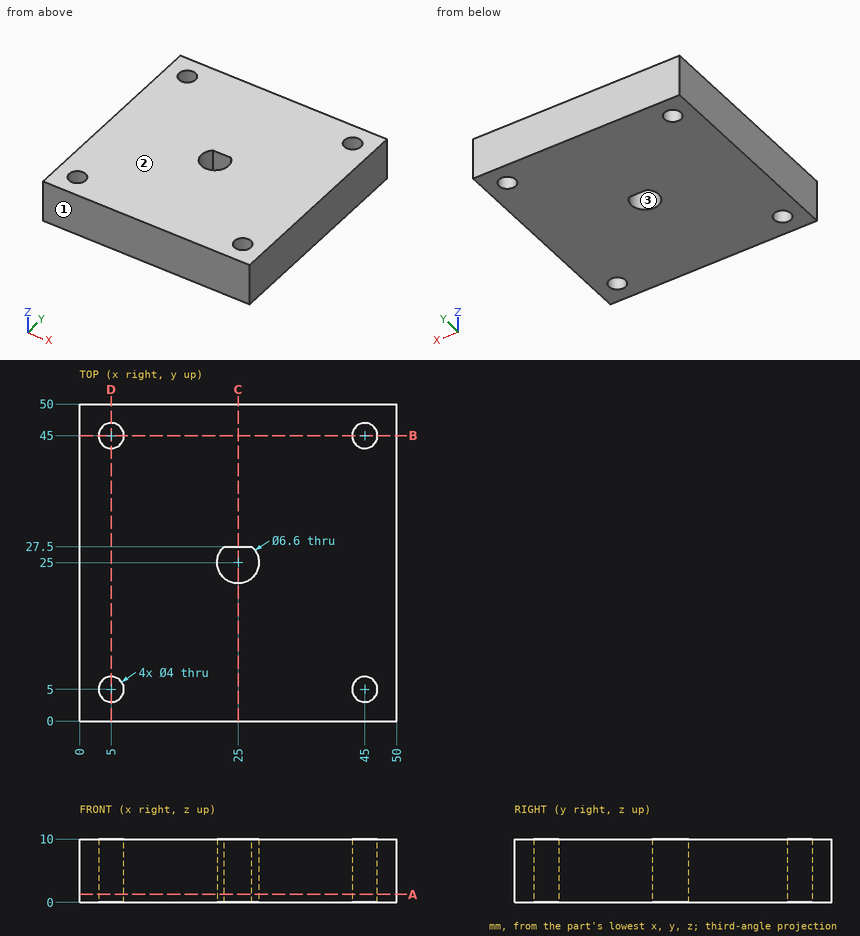
Job drawing, mm, ordinate dimensions from the low corner. One solid piece. Round coordinates to 2 decimals unless told otherwise and drop trailing zeros. Loops run counter-clockwise (first coordinate to the right, second up) from the corner with the lowest first, then second, coordinate; pieces in that order, holes last. Notation, with made-up numbers: (50.5, 8) -> (61.5, 8) arc R24 cw to (61.5, 39) -> close; hole circle Ø5 at (6.25, 44). An arc over 180 degrees is marked (long way). Use a Markdown table: item, result.
1) Drop flat-ended pins along their axis: pin 1 Ø3.5 at (x, y) = (45, 5) entering from -Z; pin 2 Ø12 at (x, y) = (26, 25.5) entering from +Z. Give the stop position or say it passes through.
The answers:
| item | result |
|---|---|
| pin 1 | passes through |
| pin 2 | stops at z = 10 |
2) Cut at C-C, the plane x = 25. List the corners of the cut face in (y, z).
The answers:
| item | result |
|---|---|
| outline | (0, 0) -> (21.7, 0) -> (21.7, 10) -> (0, 10) -> close; (27.5, 0) -> (50, 0) -> (50, 10) -> (27.5, 10) -> close |
3) Pull direction Y, two halves, no side cores. Call the marked faces 1, 2 and 3: pulls with the +Y half, pulls with the -Y half, needs draft (parallel to the pull), parting line crosses it, or undercut.
The answers:
| item | result |
|---|---|
| face 1 | pulls with the -Y half |
| face 2 | needs draft |
| face 3 | undercut |
4) Cut at A-A, the plane z = 1.25. List the corners of the cut face in (x, y).
The answers:
| item | result |
|---|---|
| outline | (0, 0) -> (50, 0) -> (50, 50) -> (0, 50) -> close; hole circle Ø4 at (5, 5); hole circle Ø4 at (5, 45); hole (22.85, 27.5) arc R3.3 ccw (long way) to (27.15, 27.5) -> close; hole circle Ø4 at (45, 5); hole circle Ø4 at (45, 45) |
5) Cut at B-B, the plane y = 45. List the corners of the cut face in (x, z).
The answers:
| item | result |
|---|---|
| outline | (0, 0) -> (3, 0) -> (3, 10) -> (0, 10) -> close; (7, 0) -> (43, 0) -> (43, 10) -> (7, 10) -> close; (47, 0) -> (50, 0) -> (50, 10) -> (47, 10) -> close |
6) Probe line 1 (Y direction, x = 5, z = 4.25); line 2 (X direction, y = 25, z = 3.5); line 3 (Y direction, x = 43.5, z = 7.25). List the from-to ranges inside material, lowest first. Write a range as [from, to].
The answers:
| item | result |
|---|---|
| line 1 | y = [0, 3], [7, 43], [47, 50] |
| line 2 | x = [0, 21.7], [28.3, 50] |
| line 3 | y = [0, 3.68], [6.32, 43.68], [46.32, 50] |
